Here's how the part is built. I have some questions about the finished solid (model axes, mm). A direction names the side the tool comes from. Coordinates: 2 decimals unless noted, no trailing zeros. Write each loop counter-clockwise with the first axis right and the second up, starting at its lowest first coordinate (ties: lowest second). Pieces come first, ordered by that corner, then holes. Notation, with made-up numbers: (66, 18) - (102, 18) arc R10 cw to (102, 27) - close; hole circle Ø5 at (27, 17). An arc over 180 degrees is marked (long way). Answer in a Markdown table with one row per item. Add a question column.
Item 1: Imagine slicing it at A-A (x = 0). Please give me the cut outline in (y, z), plus the area to 3 significant figures.
Item 2: Which directions (+Z, -Z, +X, -X, +Y, -Y) give clear straight access to the entire face, cutting with the end or side of a thin tool? Please do faces 1 (the face through (-0.54, -2.44, 16.52)), 2 (the face through (0, 2, 24)).
Item 3: I'm going to push flat-ended pins straight in: pin 1 (1 mm diameter, centred on x = -1, z = 17.5, fed in from -Y); pin 2 (1 mm diameter, centred on y = 1.5, z = 29, fed in from -X); pin 3 (2 mm diameter, centred on x = -1.5, z = 23.5, fed in from +Y). Where does each tip first touch, or does it pass through?
Item 4: If I drill on probe 1 along Z at (x, y) = (-0.1, 2.25); probe 2 along Z at (x, y) = (-2, 0.1); probe 3 along X at (y, z) = (1.95, 27), over which ranges is the centre line in solid material (lowest first)? Write a range as from..to.
Item 5: Imagine slicing it at B-B (z = 22.5). Please give me the cut outline in (x, y).
from build123d import *

# Parameters (mm, degrees)
SKETCH_1_R          = 2.5
EXTRUDE_5_DEPTH     = 34
CUT_EXTRUDE_START   = -20
CUT_EXTRUDE_2_DEPTH = 20
CHAMFER_2_SIZE      = 0.5


with BuildPart() as part:
    # 草图1 → 凸台-拉伸5 (new body)
    with BuildSketch(Plane.XY):
        Circle(SKETCH_1_R)
    extrude(amount=EXTRUDE_5_DEPTH)

    # 草图4 → 切除-拉伸2 (cut)
    with BuildSketch(Plane.XY.offset(34).offset(CUT_EXTRUDE_START)):
        with BuildLine():
            Line((-1.5, 2), (1.5, 2))
            ThreePointArc((1.5, 2), (0, 2.5), (-1.5, 2))
        make_face()
    extrude(amount=CUT_EXTRUDE_2_DEPTH, mode=Mode.SUBTRACT)

    # 倒角2
    chamfer_2_edges = [part.edges().sort_by_distance(p)[0] for p in [
        (-1.118033989, -2.236067977, 34),
        (0, 2, 34),
    ]]
    chamfer(chamfer_2_edges, length=CHAMFER_2_SIZE - 0.0001)  # a hair under: the kernel refuses the full size


solid = part.part
Here are the results:
| question | item | result |
|---|---|---|
| 1 | outline | (-2.5, 0) - (2.5, 0) - (2.5, 14) - (2, 14) - (2, 33.5) - (1.5, 34) - (-2, 34) - (-2.5, 33.5) - close |
| 1 | area | 160 mm2 |
| 2 | face 1 | +Z, -Z |
| 2 | face 2 | +Z, +X, -X, +Y |
| 3 | pin 1 | stops at y = -2.45 |
| 3 | pin 2 | stops at x = -2.29 |
| 3 | pin 3 | stops at y = 2 |
| 4 | probe 1 | z = 0..14 |
| 4 | probe 2 | z = 0..34 |
| 4 | probe 3 | x = -1.56..1.56 |
| 5 | outline | (-1.5, 2) arc R2.5 ccw (long way) to (1.5, 2) - close |
